The model under review builds one solid part; all positions refer to its coordinate system, in mm. Face numbers are marked on the shaded views. A direction names the side the tool comes from. Round coordinates to 2 decimals unless told otherwise and drop trailing zeros. Write each loop counter-clockwise with the first axis right and the second up, starting at its lowest first coordinate (ties: lowest second). Pieces come first, ordered by that corner, then holes. Notation, with made-up numbers: (-32.75, 56) - (-9.75, 56) arc R23 cw to (-9.75, 69) - close; hole circle Ø8 at (89.5, 49). An arc over 180 degrees is marked (long way). Use one line per item in the form item = value.
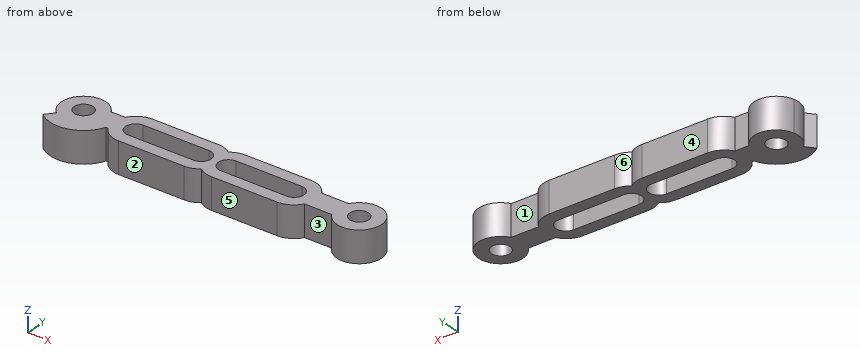
from build123d import *

# Parameters (mm, degrees)
SKETCH_1_R      = 1.7
EXTRUDE_1_DEPTH = 5.6


with BuildPart() as part:
    # Эскиз1 → Бобышка-Вытянуть1 (new body)
    with BuildSketch(Plane.XY):
        with BuildLine():
            Line((0, 4), (12, 4))
            ThreePointArc((12, 4), (13.324764885, 3.774254628), (14.5, 3.122498999))
            ThreePointArc((14.5, 3.122498999), (15.675235115, 3.774254628), (17, 4))
            Line((17, 4), (29, 4))
            ThreePointArc((29, 4), (31, 3.464101615), (32.464101615, 2))
            Line((32.464101615, 2), (37.464101615, 2))
            ThreePointArc((37.464101615, 2), (44.92820323, 0), (37.464101615, -2))
            Line((37.464101615, -2), (32.464101615, -2))
            ThreePointArc((32.464101615, -2), (31, -3.464101615), (29, -4))
            Line((29, -4), (17, -4))
            ThreePointArc((17, -4), (15.675235115, -3.774254628), (14.5, -3.122498999))
            ThreePointArc((14.5, -3.122498999), (13.324764885, -3.774254628), (12, -4))
            Line((12, -4), (0, -4))
            ThreePointArc((0, -4), (-2, -3.464101615), (-3.464101615, -2))
            Line((-3.464101615, -2), (-3.843145751, -2))
            ThreePointArc((-3.843145751, -2), (-7.906039139, -5.784400468), (-13.333929304, -4.615299133))
            Line((-13.333929304, -4.615299133), (-12.05595287, -3.076866089))
            ThreePointArc((-12.05595287, -3.076866089), (-13.289295027, -1.281110144), (-13.398667792, 0.894644872))
            ThreePointArc((-13.398667792, 0.894644872), (-10.093855563, 3.955671317), (-6.035898385, 2))
            Line((-6.035898385, 2), (-3.843145751, 2))
            Line((-3.843145751, 2), (-3.464101615, 2))
            ThreePointArc((-3.464101615, 2), (-2, 3.464101615), (0, 4))
        make_face()
        with Locations((40.92820323, 0)):
            Circle(SKETCH_1_R, mode=Mode.SUBTRACT)
        with Locations((-9.5, 0)):
            Circle(SKETCH_1_R, mode=Mode.SUBTRACT)
        with BuildLine():
            Line((0, 1.8), (12, 1.8))
            ThreePointArc((12, 1.8), (13.8, 0), (12, -1.8))
            Line((12, -1.8), (0, -1.8))
            ThreePointArc((0, -1.8), (-1.8, 0), (0, 1.8))
        make_face(mode=Mode.SUBTRACT)
        with BuildLine():
            Line((17, 1.8), (29, 1.8))
            ThreePointArc((29, 1.8), (30.8, 0), (29, -1.8))
            Line((29, -1.8), (17, -1.8))
            ThreePointArc((17, -1.8), (15.2, 0), (17, 1.8))
        make_face(mode=Mode.SUBTRACT)
    extrude(amount=EXTRUDE_1_DEPTH)


solid = part.part
(1) Add section A-A on x = -9.5. Write out the cut boundary in (y, z), then the cut area to 3 significant figures.
Geometry results:
outline = (-6, 0) - (-1.7, 0) - (-1.7, 5.6) - (-6, 5.6) - close; (1.7, 0) - (4, 0) - (4, 5.6) - (1.7, 5.6) - close
area = 37.0 mm2
(2) Add section D-D on x = 31.5. Write out the cut boundary in (y, z).
Geometry results:
outline = (-3.12, 0) - (3.12, 0) - (3.12, 5.6) - (-3.12, 5.6) - close
(3) Add section C-C on z = 1.35. Count the separate pieces of the cut face and the enclosed holes in it, then the cut area to 3 significant figures.
Geometry results:
separate_pieces = 1
enclosed_holes = 4
area = 298 mm2
(4) The part is to be moulded in two halves that separate along X. For the marked faces 1 and 2, say which applies: +X half, -X half, draft (parallel to the pull), parting line (faces both ways), or undercut.
Geometry results:
face_1 = undercut
face_2 = draft
(5) Insertion check: P1, Ø1.3, axis at x = -4.5, z = 2.5, coming from the +Y side; P2, Ø4, axis at x = 14.5, y = -3.5, coming from the +Z side; P3, Ø3, axis at x = -9.5, y = 0, coming from the +Z side; P4, Ø3, axis at x = 3.5, z = 4, coming from the -Y side. Each pin has a flat end and moves straight along its axis. Give the tip position at first contact, or say it passes through.
Geometry results:
P1 = 2
P2 = 5.6
P3 = through
P4 = -4
(6) To check wall thickness, follow L1, parallel to Y at x = -9.5, z = 4.15; L2, parallel to Y at x = 12, z = 3.1; L3, parallel to X at y = 3.5, z = 0.6. State the ranges of each line that lie inside material, in increasing order.
Geometry results:
L1 = -6 to -1.7, 1.7 to 4
L2 = -4 to -1.8, 1.8 to 4
L3 = -11.44 to -7.56, -1.94 to 13.94, 15.06 to 30.94, 38.99 to 42.86
(7) Add section B-B on y = 0. Write out the cut boundary in (x, z).
Geometry results:
outline = (-13.5, 0) - (-11.2, 0) - (-11.2, 5.6) - (-13.5, 5.6) - close; (-7.8, 0) - (-1.8, 0) - (-1.8, 5.6) - (-7.8, 5.6) - close; (13.8, 0) - (15.2, 0) - (15.2, 5.6) - (13.8, 5.6) - close; (30.8, 0) - (39.23, 0) - (39.23, 5.6) - (30.8, 5.6) - close; (42.63, 0) - (44.93, 0) - (44.93, 5.6) - (42.63, 5.6) - close
(8) Machinability: for the marked faces 3, 4, 5 and 6, which of the approach directions +Z, -Z, +X, -X, +Y, -Y give a long, thin tool a straight path to every point of the face, cutting with its end or side? Answer none if there is none.
Geometry results:
face_3 = +Z, -Z, -Y
face_4 = +Z, -Z, +X, -X, +Y
face_5 = +Z, -Z, +X, -Y
face_6 = +Z, -Z, +Y
